```python
from build123d import *

# Parameters (mm, degrees)
F0_R     = 1.25
F1_DEPTH = 5
F2_W     = 40
F2_H     = 30
F3_DEPTH = 5
F4_SIZE2 = 2.6794919243
F4_SIZE  = 10
F5_DEPTH = 5
F6_R     = 1.5
F7_DEPTH = 3


with BuildPart() as f1:
    # F0 (on Top) → F1 (new body)
    with BuildSketch(Plane.XY):
        Circle(F0_R)
    extrude(amount=F1_DEPTH)

    # F2 (on face) → F3 (join)
    with BuildSketch(Plane.XY.offset(5)):
        Rectangle(F2_W, F2_H)
    extrude(amount=F3_DEPTH)

    # F4
    f4_edges = [f1.edges().sort_by_distance(p)[0] for p in [
        (0, 15, 10),
    ]]
    f4_side = f1.faces().sort_by_distance((0, 0, 10))[0]
    chamfer(f4_edges, length=F4_SIZE, length2=F4_SIZE2, reference=f4_side)

    # F5 (cut): a face of the model
    f5_faces = [f1.faces().sort_by_distance(p)[0] for p in [
        (0, 0, 0),
    ]]
    extrude(f5_faces, amount=-F5_DEPTH, mode=Mode.SUBTRACT)

    # F6 (on face) → F7 (cut)
    with BuildSketch(Plane(origin=(0, 0, 5), x_dir=(1, 0, 0), z_dir=(0, 0, -1))):
        Circle(F6_R)
    extrude(amount=-F7_DEPTH, mode=Mode.SUBTRACT)


solid = f1.part
```
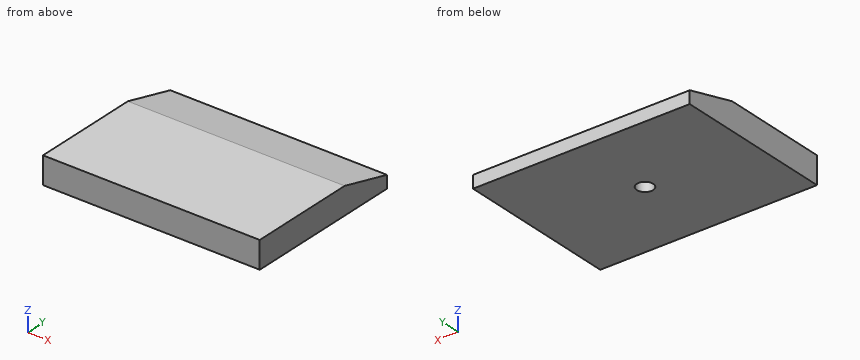
Could you check a few things on this model? Use its own coordinates, in mm. Round coordinates to 2 decimals unless told otherwise and drop trailing zeros. Write each loop counter-clockwise with the first axis right and the second up, starting at its lowest first coordinate (ties: lowest second). Pieces come first, ordered by that corner, then holes.
(1) Suppose I cut it at C-C on x = 5.5. Write out the boundary of the cut face in (y, z).
Findings below:
outline: (-15, 5) - (15, 5) - (15, 7.32) - (5, 10) - (-15, 10) - close
(2) For pin 1 (10 mm diameter, centred on x = -3.5, y = 11.5, fed in from +Z); pin 2 (2.5 mm diameter, centred on x = 0.5, y = 0.5, fed in from -Z), each with a flat end and sliding along its axis, tell me the tip position at first contact or that it passes through.
Findings below:
pin 1: stops at z = 9.6
pin 2: stops at z = 5
(3) Suppose I cut it at A-A on x = 0. Write out the boundary of the cut face in (y, z), and give its area (3 significant figures).
Findings below:
outline: (-15, 5) - (-1.5, 5) - (-1.5, 8) - (1.5, 8) - (1.5, 5) - (15, 5) - (15, 7.32) - (5, 10) - (-15, 10) - close
area: 128 mm2
(4) Suppose I cut it at D-D on z = 8.9. Write out the boundary of the cut face in (x, y).
Findings below:
outline: (-20, -15) - (20, -15) - (20, 9.11) - (-20, 9.11) - close
(5) If I drill on probe 1 along Y at (x, z) = (0, 6.25); probe 2 along X at (y, z) = (0, 6.9); probe 3 along X at (y, z) = (1, 6.5), over which ranges is the centre line in solid material (lowest first)?
Findings below:
probe 1: y = -15 to -1.5, 1.5 to 15
probe 2: x = -20 to -1.5, 1.5 to 20
probe 3: x = -20 to -1.12, 1.12 to 20
(6) Suppose I cut it at B-B on y = 0. Write out the boundary of the cut face in (x, z), and give its area (3 significant figures).
Findings below:
outline: (-20, 5) - (-1.5, 5) - (-1.5, 8) - (1.5, 8) - (1.5, 5) - (20, 5) - (20, 10) - (-20, 10) - close
area: 191 mm2
